The model under review builds one solid part; all positions refer to its coordinate system, in mm. Coordinates: 2 decimals unless noted, no trailing zeros. Loops run counter-clockwise (first coordinate to the right, second up) from the corner with the lowest first, then second, coordinate; pieces in that order, holes last. Notation, with made-up numbers: M 61.5,-0.5 L 82.5,-0.5 A25 cw 82.5,24.5 Z; hole C 42.5,89 d2. An arc over 180 degrees is marked long. Write item = value, one per line. Start each with the question number.
Q1. We need section B-B on y = 11.5. Give the boundary of the cut face in (x, z), and give its area (3 significant figures).
Q2. Clearance check with flat-ended pins moving along their axes: pin 1 Ø0.6 at (x, z) = (0, -5.5) entering from -Y; pin 2 Ø2.5 at (x, z) = (0, 2.5) entering from +Y; pin 3 Ø1 at (y, z) = (3, 6) entering from +X; pin 4 Ø1 at (x, z) = (0, 2.5) entering from +Y. State where each tip first meets the part, or that it passes through.
Q3. Wall thickness on probe 1 along Z at (x, y) = (0, 1.9); probe 2 along Z at (x, y) = (0, 10.25); probe 3 along X at (y, z) = (4, 0.5): over which ranges is each line inside the solid? List them lowest first.
Q4. We need section A-A on y = 2.5. Give the boundary of the cut face in (x, z), and give its area (3 significant figures).
Q5. We need section C-C on z = -2.5. Give the boundary of the cut face in (x, y), and give its area (3 significant figures).
Q6. We need section D-D on z = -8.25. Give the boundary of the cut face in (x, y), and give its area (3 significant figures).
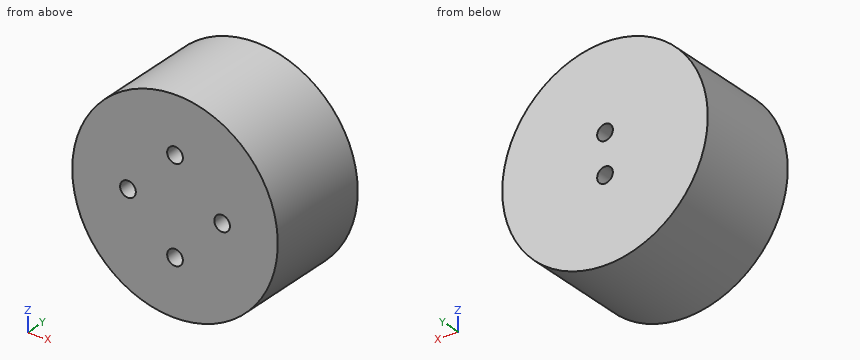
Autodesk Inventor part; units mm, degrees
ref_plane "YZ Plane" through (0, 0, 0) normal (1, 0, 0) x (0, 1, 0)
ref_plane "XZ Plane" through (0, 0, 0) normal (0, 1, 0) x (-1, 0, 0)
ref_plane "XY Plane" through (0, 0, 0) normal (0, 0, 1) x (1, 0, 0)
sketch "Sketch1" plane through (0, 0, 0) normal (0, 1, 0) x (-1, 0, 0)
  circle A0 centre (0, 0) radius 6 construction
  circle A1 centre (6, 0) radius 1
  circle A2 centre (0, 6) radius 1
  circle A3 centre (-6, 0) radius 1
  circle A4 centre (0, -6) radius 1
  circle A5 centre (0, 0) radius 13.1
  dimension "d0" = 12
  dimension "d1" = 2
  dimension "d2" = 2
  dimension "d3" = 2
  dimension "d4" = 2
  dimension "d10" = 26.2
extrude "Extrusion1" add sketch "Sketch1" along normal blind 6
sketch "Sketch2" plane through (0, 6, 0) normal (0, 1, 0) x (1, 0, 0)
  circle A0 centre (0, 0) radius 13.1
  circle A1 centre (0, 0) radius 2.5 construction
  circle A2 centre (0, -2.5) radius 1
  circle A3 centre (0, 2.5) radius 1
  dimension "d7" = 5
  dimension "d8" = 2
  dimension "d9" = 2
extrude "Extrusion2" add sketch "Sketch2" along normal blind 7.7
properties part number "motor_subsitude"
Returned:
q1.outline = C 0,0 d26.2; hole C 0,-2.5 d2; hole C 0,2.5 d2
q1.area = 533 mm^2
q2.pin_1 = 6
q2.pin_2 = 13.7
q2.pin_3 = 11.89
q2.pin_4 = 6
q3.probe_1 = -13.1 to -7, -5 to 5, 7 to 13.1
q3.probe_2 = -13.1 to -3.5, -1.5 to 1.5, 3.5 to 13.1
q3.probe_3 = -13.09 to -6.87, -5.13 to 5.13, 6.87 to 13.09
q4.outline = C 0,0 d26.2; hole C -6,0 d2; hole C 0,-6 d2; hole C 0,6 d2; hole C 6,0 d2
q4.area = 527 mm^2
q5.outline = M -12.86,0 L 12.86,0 L 12.86,13.7 L 1,13.7 L 1,6 L -1,6 L -1,13.7 L -12.86,13.7 Z
q5.area = 337 mm^2
q6.outline = M -10.18,0 L 10.18,0 L 10.18,13.7 L -10.18,13.7 Z
q6.area = 279 mm^2
